For this review, use the dimensioned drawing (mm, ordinates from the lowest corner) and the shaded views. A direction names the side the tool comes from. Coordinates: 2 decimals unless noted, no trailing zeros. Order: outer loops, then holes, each group sorted by start corner. A loop starts at its lowest first (then second) coordinate and runs counter-clockwise, first axis right, second up. Notation, with made-up numbers: M -33,13 L -18,13 A17 ccw -18,21 Z; hole C -7,88 d9. An arc over 180 degrees is marked long. Answer in a Markdown table with one row per item.
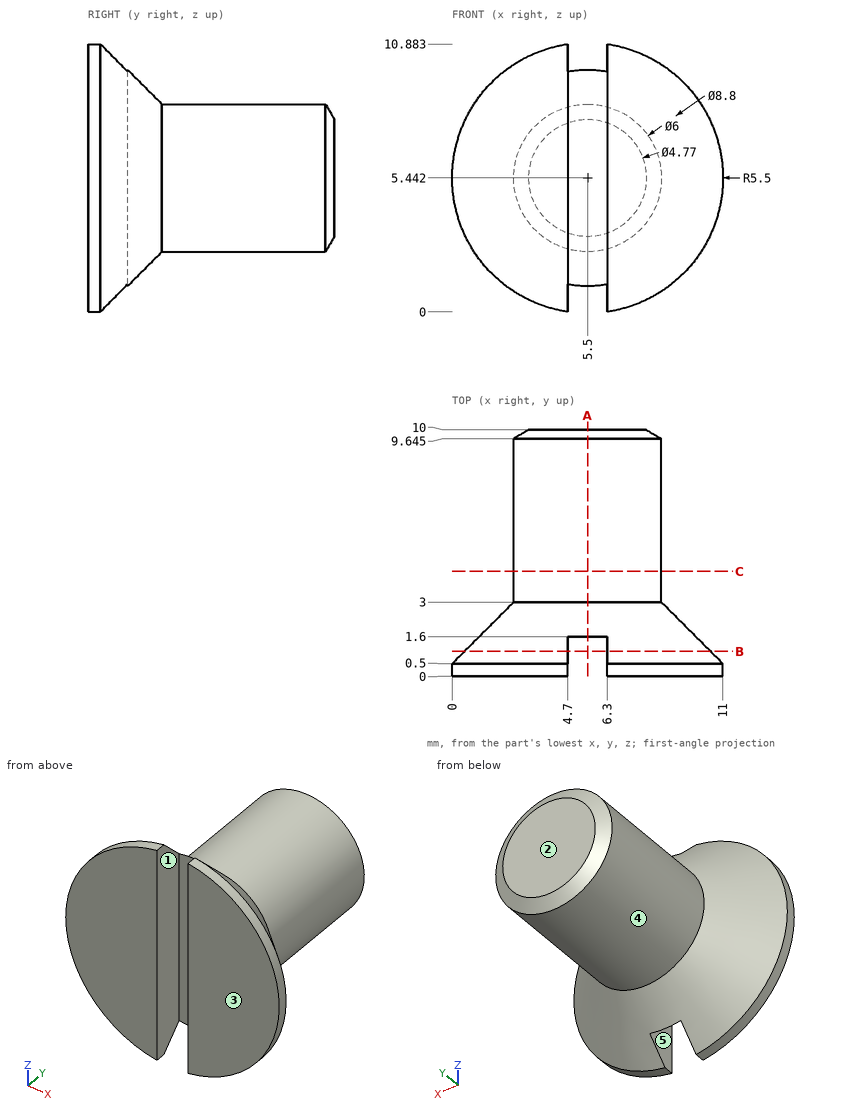
(1) Add section B-B, the plane y = 1. Give the boundary of the cut face in (x, z) (1 decimal).
Return value:
| item | result |
|---|---|
| outline | M 4.7,0.5 L 4.7,10.4 A5 ccw Z; M 6.3,0.5 A5 ccw 6.3,10.4 Z |
(2) Draft analysis for pull direction X (two halves, no side actions). For the marked faces 3, 4 and 5, state which applies: pulls with the +X half, pulls with the -X half, needs draft (parallel to the pull), parting line crosses it, or undercut.
Return value:
| item | result |
|---|---|
| face 3 | needs draft |
| face 4 | parting line crosses it |
| face 5 | undercut |
(3) For the marked faces 1 and 2, list the 3-axis set-ups (+Z, -Z, +X, -X, +Y, -Y) from which the entire face can be reached by the end or side of a thin tool; tool diameter is ignored.
Return value:
| item | result |
|---|---|
| face 1 | +Z, -Z, -Y |
| face 2 | +Z, -Z, +X, -X, +Y |
(4) Insertion check: pin 1 Ø1 at (x, y) = (4.5, 2.5) entering from -Z (1 decimal); pin 2 Ø0.5 at (y, z) = (1, 7.5) entering from +X; pin 3 Ø1.3 at (y, z) = (1, 6) entering from -X. Each pin has a flat end and moves straight along its axis. Give the tip position at first contact, or say it passes through.
Return value:
| item | result |
|---|---|
| pin 1 | stops at z = 1.6 |
| pin 2 | stops at x = 10.35 |
| pin 3 | stops at x = 0 |
(5) Add section A-A, the plane x = 5.5. Give the boundary of the cut face in (y, z) (1 decimal).
Return value:
| item | result |
|---|---|
| outline | M 1.6,1 L 3,2.4 L 9.6,2.4 L 10,3.1 L 10,7.8 L 9.6,8.4 L 3,8.4 L 1.6,9.8 Z |
(6) Add section C-C, the plane y = 4.25. Give the boundary of the cut face in (x, z).
Return value:
| item | result |
|---|---|
| outline | C 5.5,5.44 d6 |
(7) For line 1 along Y through (x, z) = (5.25, 7); line 2 along Z through (x, y) = (5, 6.75); line 3 along X through (y, z) = (8, 4), list the stretches that pass through material, from the lowest coordinate up. Write a range as from..to.
Return value:
| item | result |
|---|---|
| line 1 | y = 1.6..10 |
| line 2 | z = 2.48..8.4 |
| line 3 | x = 2.87..8.13 |
